Check sheet for the modelled part. Datum: model origin and axes. Units: mm. Give positions to 0.01 mm unless a question says otherwise; leave off trailing zeros. Write each loop counter-clockwise with the first axis right and the second up, starting at its lowest first coordinate (ties: lowest second). Pieces come first, ordered by that corner, then holes. Notation, with made-up numbers: (87.25, -12.75) -> (116.25, -12.75) arc R22 cw to (116.25, -6.75) -> close; hole circle Ø11 at (39, -12.75). An arc over 180 degrees is marked (long way). Use a Markdown table: item, result. Add a question column.
1. Gauge pin test, flat ends, axial feed: P1, Ø2, axis at x = 16.5, y = 3.5, coming from the +Z side; P2, Ø1.8, axis at x = -31.52, z = 26.6, coming from the -Y side; P3, Ø8, axis at x = 9, z = -24, coming from the -Y side. Record the tip position at first contact, or that the pin passes through.
2. Cross-section at C-C (z = 31). Enter the section's corners in (x, y), then the cut area to 3 significant figures.
3. Scan lines: probe 1 along Z at (x, y) = (-8.5, 2.4); probe 2 along X at (y, z) = (3.75, 44); probe 3 along X at (y, z) = (3.75, 26). Record each from-to range of solid material in increasing order. Write a range as [from, to].
4. Cross-section at B-B (x = 14). Enter the section's corners in (y, z).
5. Cross-section at A-A (y = 2.1). Enter the section's corners in (x, z) (3 decimals), then the cut area to 3 significant figures.
6. Release check for a two-part mould opening along Z. For faces 1 (the flat face through (21.348, 1.972, 37.675)), 2 (the cylindrical face through (-30.73, 1.58, 27.21)), 3 (the flat face through (-43.301, 2, 0)) record: released by +Z, released by -Z, zero draft, split by the parting line, or undercut.
from build123d import *

# Parameters (mm, degrees)
BOSS_EXTRUDE1_DEPTH                                  = 4
CSK_FOR_M1_6_COUNTERSUNK_FLAT_HEAD_SCREW_D           = 2
CSK_FOR_M1_6_COUNTERSUNK_FLAT_HEAD_SCREW_CSINK_D     = 3.6
CSK_FOR_M1_6_COUNTERSUNK_FLAT_HEAD_SCREW_CSINK_ANGLE = 90


with BuildPart() as part:
    # Sketch1 → Boss-Extrude1 (new body)
    with BuildSketch(Plane(origin=(0, 0, 0), x_dir=(1, 0, 0), z_dir=(0, 1, 0))):
        Polygon((0, 50), (-43.301270189, 25), (-43.301270189, -25), (0, -50), (43.301270189, -25), (43.301270189, 25), align=None)
    extrude(amount=BOSS_EXTRUDE1_DEPTH)

    # CSK for M1.6 Countersunk Flat Head Screw1 (through all)
    with Locations(Plane(origin=(-40.56776455, 4, -91.833285009), x_dir=(1, 0, 0), z_dir=(0, 1, 0))):
        with Locations((9.042773802, -118.436170692)):
            CounterSinkHole(CSK_FOR_M1_6_COUNTERSUNK_FLAT_HEAD_SCREW_D / 2, CSK_FOR_M1_6_COUNTERSUNK_FLAT_HEAD_SCREW_CSINK_D / 2, counter_sink_angle=CSK_FOR_M1_6_COUNTERSUNK_FLAT_HEAD_SCREW_CSINK_ANGLE)


solid = part.part
Worked answers:
| question | item | result |
|---|---|---|
| 1 | P1 | stops at z = 41.05 |
| 1 | P2 | passes through |
| 1 | P3 | stops at y = 0 |
| 2 | outline | (-32.91, 0) -> (32.91, 0) -> (32.91, 4) -> (-32.91, 4) -> close |
| 2 | area | 263 mm² |
| 3 | probe 1 | z = [-45.09, 45.09] |
| 3 | probe 2 | x = [-10.39, 10.39] |
| 3 | probe 3 | x = [-41.57, -32.95], [-30.1, 41.57] |
| 4 | outline | (0, -41.92) -> (4, -41.92) -> (4, 41.92) -> (0, 41.92) -> close |
| 5 | outline | (-43.301, -25) -> (0, -50) -> (43.301, -25) -> (43.301, 25) -> (0, 50) -> (-43.301, 25) -> close; hole circle Ø2 at (-31.525, 26.603) |
| 5 | area | 6,490 mm² |
| 6 | face 1 | released by +Z |
| 6 | face 2 | undercut |
| 6 | face 3 | zero draft |
